Here's the drawing with two shaded views (mm, measured from the low corner). I have some questions. Give positions to 0.01 mm unless a question says otherwise; leave off trailing zeros. Loops run counter-clockwise (first coordinate to the right, second up) from the corner with the lowest first, then second, coordinate; pieces in that order, holes last. Notation, with made-up numbers: (46, 34) - (76, 34) arc R21 ccw to (76, 64) - close; hole circle Ø2 at (-28, 70). An arc over 180 degrees is marked (long way). Answer as a JSON object with one key per item and string values. Group by question number.
Item 1: Suppose I cut it at B-B on x = 4. Write out the boundary of the cut face in (y, z), and give its area (3 significant figures).
Item 2: Please list where these lines run through material, in increasing order: L1, parallel to X at y = 0.6, z = 5; L2, parallel to Z at x = 21, y = 0.3; L3, parallel to X at y = 0.4, z = 8.5.
Item 3: Suppose I cut it at D-D on x = 29.5. Write out the boundary of the cut face in (y, z).
Item 4: Suppose I cut it at C-C on y = 0.4. Write out the boundary of the cut face in (x, z).
Item 5: Suppose I cut it at A-A on z = 5. Write out the boundary of the cut face in (x, y).
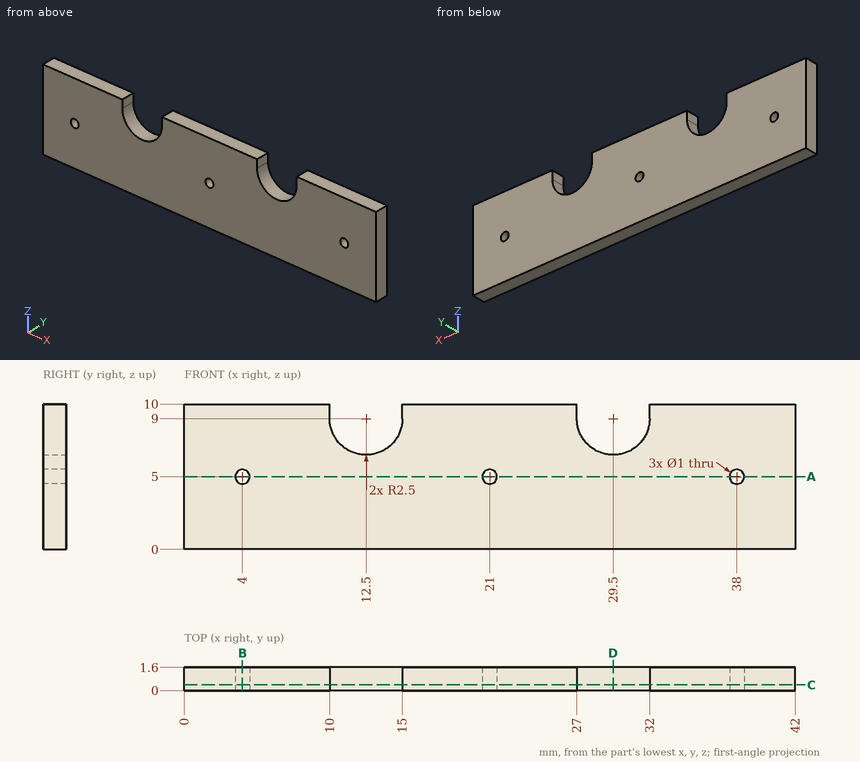
Worked out:
{
 "1": {"outline": "(0, 0) - (1.6, 0) - (1.6, 4.5) - (0, 4.5) - close; (0, 5.5) - (1.6, 5.5) - (1.6, 10) - (0, 10) - close", "area": "14.4 mm2"},
 "2": {"L1": "x = 0 to 3.5, 4.5 to 20.5, 21.5 to 37.5, 38.5 to 42", "L2": "z = 0 to 4.5, 5.5 to 10", "L3": "x = 0 to 10.05, 14.95 to 27.05, 31.95 to 42"},
 "3": {"outline": "(0, 0) - (1.6, 0) - (1.6, 6.5) - (0, 6.5) - close"},
 "4": {"outline": "(0, 0) - (42, 0) - (42, 10) - (32, 10) - (32, 9) arc R2.5 cw to (27, 9) - (27, 10) - (15, 10) - (15, 9) arc R2.5 cw to (10, 9) - (10, 10) - (0, 10) - close; hole circle Ø1 at (4, 5); hole circle Ø1 at (21, 5); hole circle Ø1 at (38, 5)"},
 "5": {"outline": "(0, 0) - (3.5, 0) - (3.5, 1.6) - (0, 1.6) - close; (4.5, 0) - (20.5, 0) - (20.5, 1.6) - (4.5, 1.6) - close; (21.5, 0) - (37.5, 0) - (37.5, 1.6) - (21.5, 1.6) - close; (38.5, 0) - (42, 0) - (42, 1.6) - (38.5, 1.6) - close"}
}
